```python
from build123d import *

# Parameters (mm, degrees)
EXTRUDE_1_DEPTH = 5
SKETCH_2_W      = 12.5
SKETCH_2_H      = 10
SKETCH_2_R      = 2.5
EXTRUDE_2_DEPTH = 5
FILLET_1_R      = 1


with BuildPart() as part:
    # 草图1 → 凸台-拉伸1 (new, symmetric)
    with BuildSketch(Plane.XY):
        with BuildLine():
            Line((16.45, 0), (22.5, 0))
            Line((22.5, 0), (22.5, 28.066706708))
            Line((22.5, 28.066706708), (-22.5, 28.066706708))
            Line((-22.5, 28.066706708), (-22.5, 0))
            Line((-22.5, 0), (-16.45, 0))
            ThreePointArc((-16.45, 0), (0, 16.45), (16.45, 0))
        make_face()
    extrude(amount=EXTRUDE_1_DEPTH, both=True)

    # 草图2 → 凸台-拉伸2 (add)
    # profile 1 of 2: a face of its own
    with BuildSketch(Plane.XZ):
        with Locations((-28.75, 0)):
            Rectangle(SKETCH_2_W, SKETCH_2_H)
        with Locations((-30, 0)):
            Circle(SKETCH_2_R, mode=Mode.SUBTRACT)
    # profile 2 of 2: a face of its own
    with BuildSketch(Plane.XZ):
        with Locations((28.75, 0)):
            Rectangle(SKETCH_2_W, SKETCH_2_H)
        with Locations(Location((30, 0, 0), (0, 0, 180))):
            Circle(SKETCH_2_R, mode=Mode.SUBTRACT)
    extrude(amount=-EXTRUDE_2_DEPTH)

    # 圆角1
    fillet_1_edges = [part.edges().sort_by_distance(p)[0] for p in [
        (22.5, 5, 0),
        (-22.5, 5, 0),
    ]]
    fillet(fillet_1_edges, radius=FILLET_1_R)


solid = part.part
```
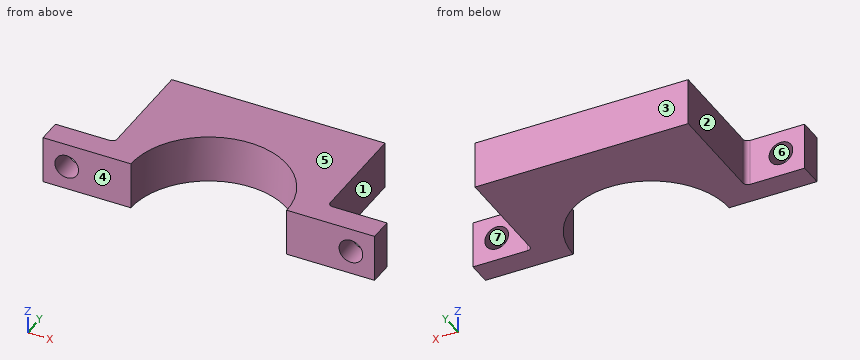
CAD build for the part. Positions are in the model's coordinates, mm. Face numbers are marked on the shaded views. A direction names the side the tool comes from. Coordinates: 2 decimals unless noted, no trailing zeros. Write each loop counter-clockwise with the first axis right and the second up, starting at its lowest first coordinate (ties: lowest second). Pieces come first, ordered by that corner, then holes. Notation, with made-up numbers: (35.25, -22) -> (65.25, -22) arc R16 cw to (65.25, -13) -> close; hole circle Ø2 at (-26.75, 44). An arc over 180 degrees is marked (long way). Return JSON: item names as keys, results as strings. Group by question number.
Q1. Cut at B-B, the plane y = 7.5. Give the cut face in (x, z), then the cut area to 3 significant figures.
Q2. Drill centre lines: line 1 (Z direction, x = 30, y = 1.75); line 2 (X direction, y = 25, z = -2); line 3 (Y direction, x = 0, z = 1.5). Where is each one in solid material? Low to high.
Q3. Cut at D-D, the plane y = 21.5. Give the cut face in (x, z), then the cut area to 3 significant figures.
Q4. Which spindle directions (+Z, -Z, +X, -X, +Y, -Y) get a long thin tool onto all of the face, cutting with end or side? Do the marked faces 1, 2 and 3. Say none if no direction does.
Q5. Pull direction Z, two halves, no side cores. Call the marked faces 4, 5, 6 and 7: released by +Z, released by -Z, zero draft, split by the parting line, or undercut.
Q6. Cut at A-A, the plane x = 30. Give the cut face in (y, z), then the cut area to 3 significant figures.
Q7. Cut at C-C, the plane x = 0. Give the cut face in (y, z), then the cut area to 3 significant figures.
Q8. Flat gauge pin, fed straight in: pin 1 (3 mm diameter, centred on x = -27, z = 1.5, fed in from +Y). Where does the tip first touch, or does it go through?
Returned:
{
 "1": {"outline": "(-22.5, -5) -> (-14.64, -5) -> (-14.64, 5) -> (-22.5, 5) -> close; (14.64, -5) -> (22.5, -5) -> (22.5, 5) -> (14.64, 5) -> close", "area": "157 mm2"},
 "2": {"line 1": "z = -5 to -2.5, 2.5 to 5", "line 2": "x = -22.5 to 22.5", "line 3": "y = 16.45 to 28.07"},
 "3": {"outline": "(-22.5, -5) -> (22.5, -5) -> (22.5, 5) -> (-22.5, 5) -> close", "area": "450 mm2"},
 "4": {"face 1": "+Z, -Z, +X, +Y", "face 2": "+Z, -Z, -X, +Y", "face 3": "+Z, -Z, +X, -X, +Y"},
 "5": {"face 4": "zero draft", "face 5": "released by +Z", "face 6": "undercut", "face 7": "undercut"},
 "6": {"outline": "(0, -5) -> (5, -5) -> (5, -2.5) -> (0, -2.5) -> close; (0, 2.5) -> (5, 2.5) -> (5, 5) -> (0, 5) -> close", "area": "25.0 mm2"},
 "7": {"outline": "(16.45, -5) -> (28.07, -5) -> (28.07, 5) -> (16.45, 5) -> close", "area": "116 mm2"},
 "8": {"pin 1": "stops at y = 5"}
}
